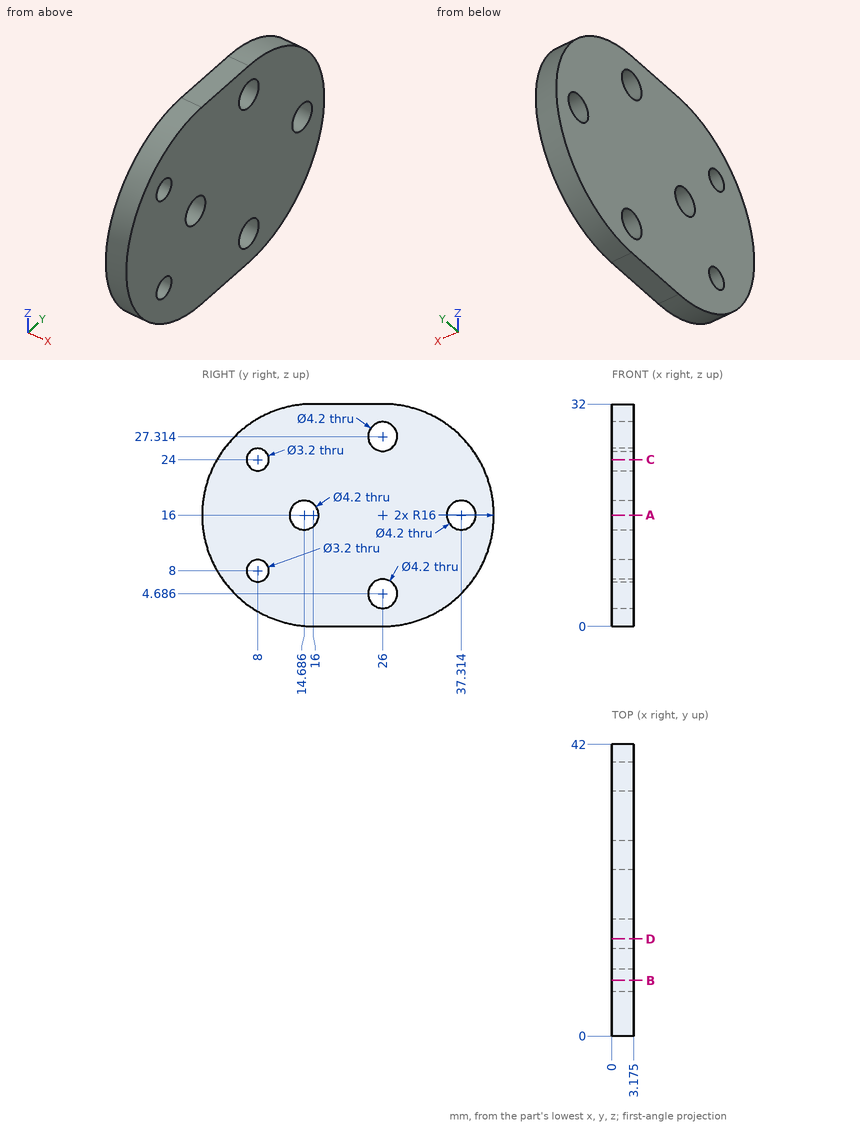
Verification items for this drawing (mm, ordinates from the low corner). Round coordinates to 2 decimals unless told otherwise and drop trailing zeros. Order: outer loops, then holes, each group sorted by start corner. A loop starts at its lowest first (then second) coordinate and runs counter-clockwise, first axis right, second up. Notation, with made-up numbers: (80.5, 70.25) -> (85.5, 70.25) arc R10 cw to (85.5, 88.25) -> close; hole circle Ø3 at (18, 12). An arc over 180 degrees is marked (long way). Use one line per item in the form item = value.
1. Cross-section at A-A, the plane z = 16. Enter the section's corners in (x, y) (1 decimal).
Working result:
outline = (0, 0) -> (3.2, 0) -> (3.2, 12.6) -> (0, 12.6) -> close; (0, 16.8) -> (3.2, 16.8) -> (3.2, 35.2) -> (0, 35.2) -> close; (0, 39.4) -> (3.2, 39.4) -> (3.2, 42) -> (0, 42) -> close
2. Cross-section at B-B, the plane y = 8. Enter the section's corners in (x, z) (1 decimal).
Working result:
outline = (0, 2.1) -> (3.2, 2.1) -> (3.2, 6.4) -> (0, 6.4) -> close; (0, 9.6) -> (3.2, 9.6) -> (3.2, 22.4) -> (0, 22.4) -> close; (0, 25.6) -> (3.2, 25.6) -> (3.2, 29.9) -> (0, 29.9) -> close
3. Go/stop test with a flat-tipped pin: pin 1 (1.5 mm diameter, centred on x = 2, z = 26, fed in from -Y) (1 decimal). Record where the tip stops, or that it passes through.
Working result:
pin_1 = 2.9
4. Scan lines: line 1 along Y through (x, z) = (2.2, 16); line 2 along Z through (x, y) = (0.3, 27); line 3 along Y through (x, z) = (2.5, 8). Record each from-to range of solid material in increasing order. Write a range as from..to.
Working result:
line_1 = 0..12.59, 16.79..35.21, 39.41..42
line_2 = 0.03..2.84, 6.53..25.47, 29.16..31.97
line_3 = 2.14..6.4, 9.6..39.86
5. Cross-section at C-C, the plane z = 24. Enter the section's corners in (x, y) (1 decimal).
Working result:
outline = (0, 2.1) -> (3.2, 2.1) -> (3.2, 6.4) -> (0, 6.4) -> close; (0, 9.6) -> (3.2, 9.6) -> (3.2, 39.9) -> (0, 39.9) -> close
6. Cross-section at D-D, the plane y = 14. Enter the section's corners in (x, z) (1 decimal).
Working result:
outline = (0, 0.1) -> (3.2, 0.1) -> (3.2, 14) -> (0, 14) -> close; (0, 18) -> (3.2, 18) -> (3.2, 31.9) -> (0, 31.9) -> close
